```python
from build123d import *

# Parameters (mm, degrees)
F0_R     = 50
F1_DEPTH = 25
F2_R     = 52
F2_R_2   = 50
F3_DEPTH = 10
F5_T     = -1.5
F6_R     = 33.5
F6_R_2   = 31.5
F7_DEPTH = 5
F8_R     = 1


# Not quite as in the source:
# - a feature of the source that left no trace in its solid (it failed there, or was rolled back) is left out


with BuildPart() as f1:
    # F0 (on Front) → F1 (new body)
    with BuildSketch(Plane.XZ):
        Circle(F0_R)
    extrude(amount=F1_DEPTH)

    # F2 (on face) → F3 (join)
    with BuildSketch(Plane.XZ.offset(25)):
        Circle(F2_R)
        Circle(F2_R_2, mode=Mode.SUBTRACT)
        Circle(F2_R_2)
    extrude(amount=F3_DEPTH)

    # F5
    f5_openings = [f1.faces().sort_by_distance(p)[0] for p in [
        (0, 0, 0),
    ]]
    offset(amount=F5_T, openings=f5_openings, kind=Kind.INTERSECTION)

    # F6 (on face) → F7 (join)
    with BuildSketch(Plane(origin=(0, -33.5, 0), x_dir=(-1, 0, 0), z_dir=(0, 1, 0))):
        Circle(F6_R)
        Circle(F6_R_2, mode=Mode.SUBTRACT)
    extrude(amount=F7_DEPTH)

    # F8
    f8_edges = [f1.edges().sort_by_distance(p)[0] for p in [
        (31.5, -28.5, 0),
        (-52, -35, 0),
        (-50, 0, 0),
    ]]
    fillet(f8_edges, radius=F8_R)


solid = f1.part
```
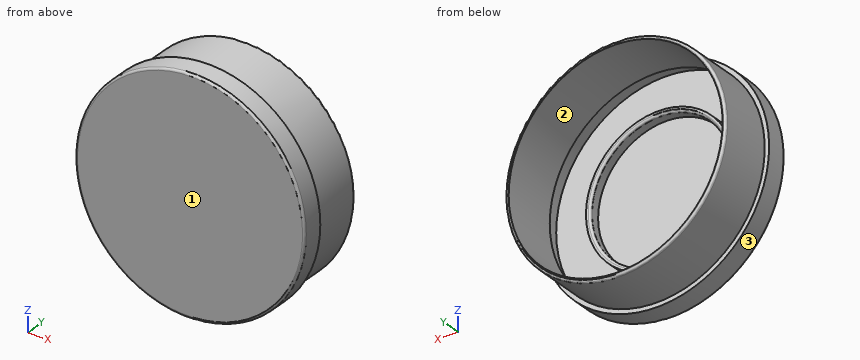
Source: CAD feature listing. Evaluate the final solid. Frame: model axes, mm. Face numbers are marked on the shaded views. Coordinates: 2 decimals unless noted, no trailing zeros. Order: outer loops, then holes, each group sorted by start corner. A loop starts at its lowest first (then second) coordinate and runs counter-clockwise, first axis right, second up. Notation, with made-up numbers: (89.25, -4) - (147.25, -4) arc R16 ccw to (147.25, 8) - close; hole circle Ø9 at (69, 71.5). An arc over 180 degrees is marked (long way). One line per item, written item: value.
1) Ray query, line 1 (Z direction, x = 0, y = -29.5); line 2 (Z direction, x = 0, y = -12); line 3 (X direction, y = -4.5, z = -1). Return the intervals inside material, ascending. Write a range as [from, to].
Computed values:
line 1: z = [-52, -50.5], [-33.5, -31.5], [31.5, 33.5], [50.5, 52]
line 2: z = [-50, -48.5], [48.5, 50]
line 3: x = [-49.99, -48.49], [48.49, 49.99]
2) Contact query for flat-ended pins moving along their axis: pin 1 (1.5 mm diameter, centred on y = -25, z = 7, fed in from -X); pin 2 (1.5 mm diameter, centred on x = -25.5, z = 23, fed in from +Y); pin 3 (8 mm diameter, centred on x = 11, y = -12.5, fed in from +Z). Output: stop coordinate, or through.
Computed values:
pin 1: stops at x = -51.62
pin 2: stops at y = -33.5
pin 3: stops at z = 49.51
3) Mould query, pull axis Z, two halves, no side actions, for the marked faces 1, 2 and 3. Classes: released by +Z, released by -Z, zero draft, split by the parting line, or undercut.
Computed values:
face 1: zero draft
face 2: undercut
face 3: split by the parting line
4) Cut plane C-C on y = -9.5. Output: boundary loops of the cut face in (x, z), plus the area to 3 significant figures.
Computed values:
outline: circle Ø100 at (0, 0); hole circle Ø97 at (0, 0)
area: 464 mm^2
